Verification items for the finished model (mm, model axes). A direction names the side the tool comes from. Coordinates: 2 decimals unless noted, no trailing zeros. Order: outer loops, then holes, each group sorted by start corner. A loop starts at its lowest first (then second) coordinate and runs counter-clockwise, first axis right, second up. Notation, with made-up numbers: M -26,29 L -19,29 A23 cw -19,46 Z; hole C -9,-37.5 d7. An arc over 180 degrees is marked long. Return JSON: item names as keys, results as strings. Group by question number.
Q1. Section check A-A, the plane x = -41. Enter the section's corners in (y, z), then the cut area to 3 significant figures.
Q2. Go/stop test with flat-tipped pins: pin 1 Ø5 at (x, y) = (-8, 22) entering from -Z; pin 2 Ø23 at (x, y) = (-11.5, 6.5) entering from +Z; pin 3 Ø1.5 at (x, y) = (-33.5, 4) entering from +Z. Record where each tip stops, or that it passes through.
Q3. Section check C-C, the plane x = -19. Enter the section's corners in (y, z).
Q4. Mould release check, pull along Z, two halves, no side actions. Record for faces 1 (the face through (0, 7, -10)), 2 (the face through (-41, 0, -25)), 3 (the face through (-59, 17, 0)): pulls with the +Z half, pulls with the -Z half, needs draft (parallel to the pull), parting line crosses it, or undercut.
Q5. Thickness scan on probe 1 along X at (y, z) = (-30, -0.5); probe 2 along Y at (x, z) = (-61, -4.5); probe 3 along Z at (x, y) = (-61, 0). Record the ranges inside material, lowest first.
Q6. Section check B-B, the plane y = -19. Enter the section's corners in (x, z), then the cut area to 3 significant figures.
Q7. Access from +Z, -Z, +X, -X, +Y, -Y to the whole of each face (thin tool, end or side, straight path). Record for faces 4 (the face through (-14, -22, -5)), 5 (the face through (-10, 0, -15)), 6 (the face through (-25, -35, 0)).
Q8. Section check D-D, the plane z = 8. Enter the section's corners in (x, y), then the cut area to 3 significant figures.
from build123d import *

# Parameters (mm, degrees)
F0_W        = 70
F0_H        = 30
F1_DEPTH    = 66
F3_DEPTH    = 70
F4_R        = 13
F5_DEPTH    = 71
F6_W        = 10
F6_H        = 10
F6_R        = 11
F7_DEPTH    = 70
F8_T1_DEPTH = 149.09177361
F9_T1_DEPTH = 8.9088895058
F9_T3_DEPTH = 6.9088895058


# Not quite as in the source:
# - a fillet or chamfer that OpenCascade refuses, or shapes differently, is made with other operations: its cross-section is extruded or revolved along the edge and cut away or added


with BuildPart() as f1:
    # F0 (on Right) → F1 (new body)
    with BuildSketch(Plane.YZ):
        Rectangle(F0_W, F0_H)
    extrude(amount=-F1_DEPTH)

    # F2 (on face) → F3 (join)
    with BuildSketch(Plane.XZ.offset(35)):
        with BuildLine():
            Line((-41, 15), (-21, 15))
            ThreePointArc((-21, 15), (-41, 25), (-61, 15))
            Line((-61, 15), (-41, 15))
        make_face()
        with BuildLine():
            ThreePointArc((-61, -15), (-41, -25), (-21, -15))
            Line((-21, -15), (-61, -15))
        make_face()
    extrude(amount=-F3_DEPTH)

    # F4 (on face) → F5 (cut)
    with BuildSketch(Plane.XZ.offset(35)):
        with Locations((-41, 0)):
            Circle(F4_R)
    extrude(amount=-F5_DEPTH, mode=Mode.SUBTRACT)

    # F6 (on face) → F7 (cut)
    with BuildSketch(Plane.YZ):
        with Locations((-22, 0)):
            Rectangle(F6_W, F6_H)
        Circle(F6_R)
        with Locations((22, 0)):
            Rectangle(F6_W, F6_H)
    extrude(amount=-F7_DEPTH, mode=Mode.SUBTRACT)

    # F8: fillet of radius 27.5220346111 on 2 edges, made by hand

    # F8_s2 → F8_t1 (cut)
    with BuildSketch(Plane.XZ.offset(-74.545886805)):
        with BuildLine():
            ThreePointArc((-66, -0.818354722), (-64.7202462083, 7.4765284314), (-61, 15))
            Line((-61, 15), (-66, 15))
            Line((-66, 15), (-66, -0.818354722))
        make_face()
        with BuildLine():
            ThreePointArc((-61, -15), (-64.7202462083, -7.4765284314), (-66, 0.818354722))
            Line((-66, 0.818354722), (-66, -15))
            Line((-66, -15), (-61, -15))
        make_face()
    extrude(amount=F8_T1_DEPTH, mode=Mode.SUBTRACT)

    # F9: fillet of radius 5 on 2 edges, made by hand

    # F9_s2 → F9_t1 (cut)
    with BuildSketch(Plane.XZ.offset(26.5455552471)):
        with BuildLine():
            ThreePointArc((-65.9818255238, 0.1816786841), (-65.9851273284, 0), (-65.9818255238, -0.1816786841))
            ThreePointArc((-65.9818255238, -0.1816786841), (-65.9849780634, -0.0908442999), (-65.9878306136, 0))
            ThreePointArc((-65.9878306136, 0), (-65.9849780634, 0.0908442999), (-65.9818255238, 0.1816786841))
        make_face()
    extrude(amount=F9_T1_DEPTH, mode=Mode.SUBTRACT)

    # F9_s4 → F9_t3 (cut)
    with BuildSketch(Plane.XZ.offset(10.5455552471)):
        with BuildLine():
            ThreePointArc((-65.9818255238, 0.1816786841), (-65.9851273284, 0), (-65.9818255238, -0.1816786841))
            ThreePointArc((-65.9818255238, -0.1816786841), (-65.9849780634, -0.0908442999), (-65.9878306136, 0))
            ThreePointArc((-65.9878306136, 0), (-65.9849780634, 0.0908442999), (-65.9818255238, 0.1816786841))
        make_face()
    extrude(amount=F9_T3_DEPTH, mode=Mode.SUBTRACT)


solid = f1.part
Numbers:
{
 "1": {"outline": "M -35,-25 L 35,-25 L 35,-13 L -35,-13 Z; M -35,13 L 35,13 L 35,25 L -35,25 Z", "area": "1,680 mm2"},
 "2": {"pin 1": "stops at z = -15", "pin 2": "stops at z = 17.35", "pin 3": "stops at z = 24.07"},
 "3": {"outline": "M -35,-15 L 35,-15 L 35,15 L -35,15 Z; hole M -27,-5 L -17,-5 L -17,5 L -27,5 Z; hole C 0,0 d22; hole M 17,-5 L 27,-5 L 27,5 L 17,5 Z"},
 "4": {"face 1": "needs draft", "face 2": "pulls with the -Z half", "face 3": "undercut"},
 "5": {"probe 1": "x = -65.97 to -53.99, -28.01 to 0", "probe 2": "y = -35 to -27, -17 to -10.04, 10.04 to 17, 27 to 35", "probe 3": "z = -15 to -11, 11 to 15"},
 "6": {"outline": "M -65.38,-5 A27.52 ccw -61,-15 A25 ccw -21,-15 L 0,-15 L 0,-5 L -29,-5 A13 cw -53,-5 Z; M -65.38,5 L -53,5 A13 cw -29,5 L 0,5 L 0,15 L -21,15 A25 ccw -61,15 A27.52 ccw Z", "area": "1,550 mm2"},
 "7": {"face 4": "+X, -X", "face 5": "-Z, +X, +Y, -Y", "face 6": "+Z, -Z, +X, -X, -Y"},
 "8": {"outline": "M -64.55,-35 L -51.25,-35 L -51.25,-7.55 L -64.55,-7.55 Z; M -64.55,7.55 L -51.25,7.55 L -51.25,35 L -64.55,35 Z; M -30.75,-35 L 0,-35 L 0,-7.55 L -30.75,-7.55 Z; M -30.75,7.55 L 0,7.55 L 0,35 L -30.75,35 Z", "area": "2,420 mm2"}
}
